```python
from build123d import *

# Parameters (mm, degrees)
F2_DEPTH    = 80
F3_DEPTH    = 5
F4_W        = 80
F4_H        = 3
F5_DEPTH    = 5
F6_T1_DEPTH = 89.0924813444
F6_T4_ANGLE = 180
F6_T6_ANGLE = 180
F7_T1_DEPTH = 89.0924813444
F7_T4_ANGLE = 180
F7_T6_ANGLE = 180


# Not quite as in the source:
# - a fillet or chamfer that OpenCascade refuses, or shapes differently, is made with other operations: its cross-section is extruded or revolved along the edge and cut away or added


with BuildPart() as f2:
    # F0 (on Top) → F2 (new body)
    with BuildSketch(Plane.XY):
        with BuildLine():
            Line((44.6416767532, 25), (-44.4508045912, 25))
            ThreePointArc((-44.4508045912, 25), (-69.4508045912, 0), (-44.4508045912, -25))
            Line((-44.4508045912, -25), (44.6416767532, -25))
            ThreePointArc((44.6416767532, -25), (69.6416767532, 0), (44.6416767532, 25))
        make_face()
        with BuildLine():
            Line((-45.3583232468, 19.9793996379), (-45.3583232468, 20.0206003621))
            Line((-45.3583232468, 20.0206003621), (44.6416767532, 20.0206003621))
            Line((44.6416767532, 20.0206003621), (44.6416767532, 20))
            ThreePointArc((44.6416767532, 20), (64.6365259994, -0.4538762181), (43.7341580975, -19.9793996379))
            Line((43.7341580975, -19.9793996379), (-43.5432859355, -19.9793996379))
            ThreePointArc((-43.5432859355, -19.9793996379), (-44.4508045912, -20), (-45.3583232468, -19.9793996379))
            ThreePointArc((-45.3583232468, -19.9793996379), (-64.4508045912, 0), (-45.3583232468, 19.9793996379))
        make_face(mode=Mode.SUBTRACT)
    extrude(amount=F2_DEPTH)

    # F1 (on Top) → F3 (join)
    with BuildSketch(Plane.XY):
        with BuildLine():
            Line((45.1049394906, 20), (-44.8950605094, 20))
            ThreePointArc((-44.8950605094, 20), (-64.8950605094, 0), (-44.8950605094, -20))
            Line((-44.8950605094, -20), (-39.8680716753, -20))
            Line((-39.8680716753, -20), (40.1319283247, -20))
            Line((40.1319283247, -20), (45.1049394906, -20))
            ThreePointArc((45.1049394906, -20), (65.1049394906, 0), (45.1049394906, 20))
        make_face()
    extrude(amount=F3_DEPTH)

    # F4 (on face) → F5 (join)
    with BuildSketch(Plane.XY.offset(5)):
        with Locations((0.1319283247, -1.5)):
            Rectangle(F4_W, F4_H)
    extrude(amount=F5_DEPTH)

    # F6: fillet of radius 5 on 1 edges, made by hand

    # F6_s2 → F6_t1 (cut)
    with BuildSketch(Plane.YZ.offset(-44.4508045912)):
        with BuildLine():
            ThreePointArc((-20, 80), (-23.5355339059, 78.5355339059), (-25, 75))
            Line((-25, 75), (-25, 80))
            Line((-25, 80), (-20, 80))
        make_face()
        with BuildLine():
            ThreePointArc((25, 75), (23.5355339059, 78.5355339059), (20, 80))
            Line((20, 80), (25, 80))
            Line((25, 80), (25, 75))
        make_face()
    extrude(amount=F6_T1_DEPTH, mode=Mode.SUBTRACT)

    # F6_s3 → F6_t4 (revolve, cut)
    with BuildSketch(Plane.YZ.offset(-44.4508045912)):
        with BuildLine():
            ThreePointArc((25, 75), (23.5355339059, 78.5355339059), (20, 80))
            Line((20, 80), (25, 80))
            Line((25, 80), (25, 75))
        make_face()
    revolve(axis=Axis((-44.4508045912, 0, 80), (0, 0, 1)), revolution_arc=F6_T4_ANGLE, mode=Mode.SUBTRACT)

    # F6_s5 → F6_t6 (revolve, cut)
    with BuildSketch(Plane.YZ.offset(44.6416767532)):
        with BuildLine():
            ThreePointArc((-25, 75), (-23.5355339059, 78.5355339059), (-20, 80))
            Line((-20, 80), (-25, 80))
            Line((-25, 80), (-25, 75))
        make_face()
    revolve(axis=Axis((44.6416767532, 0, 80), (0, 0, 1)), revolution_arc=F6_T6_ANGLE, mode=Mode.SUBTRACT)

    # F7: fillet of radius 5 on 5 edges, made by hand

    # F7_s2 → F7_t1 (cut)
    with BuildSketch(Plane.YZ.offset(-44.4508045912)):
        with BuildLine():
            ThreePointArc((-20, 0), (-23.5355339059, 1.4644660941), (-25, 5))
            Line((-25, 5), (-25, 0))
            Line((-25, 0), (-20, 0))
        make_face()
        with BuildLine():
            ThreePointArc((25, 5), (23.5355339059, 1.4644660941), (20, 0))
            Line((20, 0), (25, 0))
            Line((25, 0), (25, 5))
        make_face()
    extrude(amount=F7_T1_DEPTH, mode=Mode.SUBTRACT)

    # F7_s3 → F7_t4 (revolve, cut)
    with BuildSketch(Plane.YZ.offset(-44.4508045912)):
        with BuildLine():
            ThreePointArc((20, 0), (23.5355339059, 1.4644660941), (25, 5))
            Line((25, 5), (25, 0))
            Line((25, 0), (20, 0))
        make_face()
    revolve(axis=Axis((-44.4508045912, 0, 0), (0, 0, 1)), revolution_arc=F7_T4_ANGLE, mode=Mode.SUBTRACT)

    # F7_s5 → F7_t6 (revolve, cut)
    with BuildSketch(Plane.YZ.offset(44.6416767532)):
        with BuildLine():
            ThreePointArc((-20, 0), (-23.5355339059, 1.4644660941), (-25, 5))
            Line((-25, 5), (-25, 0))
            Line((-25, 0), (-20, 0))
        make_face()
    revolve(axis=Axis((44.6416767532, 0, 0), (0, 0, 1)), revolution_arc=F7_T6_ANGLE, mode=Mode.SUBTRACT)


solid = f2.part
```
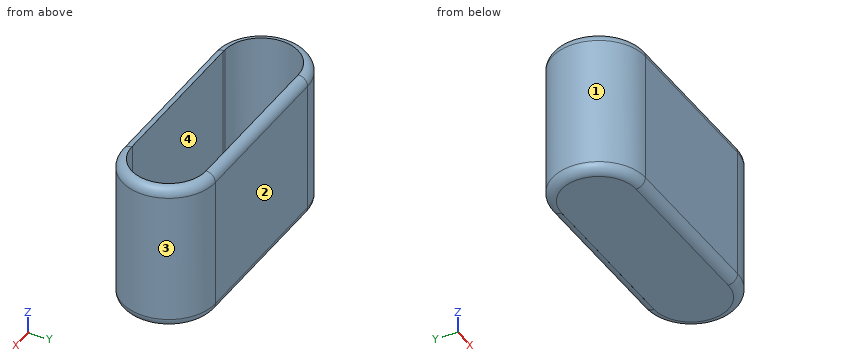
Geometry check sheet. Reference: the model listing, model coordinates, mm. Face numbers are marked on the shaded views. Coordinates: 2 decimals unless noted, no trailing zeros. Answer as a JSON object with one key per item and string values.
Q1. Scan lines: line 1 (Y direction, x = -32, z = 17.5); line 2 (Z direction, x = 12, y = -8.5); line 3 (X direction, y = -1, z = 62.5). Record each from-to range of solid material in increasing order.
Results are:
{"line 1": "y = -25 to -19.98, 20.02 to 25", "line 2": "z = 0 to 5", "line 3": "x = -69.43 to -64.43, 64.62 to 69.62"}
Q2. Depth check by flat-ended pin: pin 1 Ø5 at (y, z) = (14, 71) entering from -X; pin 2 Ø10 at (y, z) = (18, 22.5) entering from +X; pin 3 Ø2 at (y, z) = (-8.5, 44.5) entering from +X; pin 4 Ø5 at (x, z) = (46.5, 33) entering from -Y. Enter the tip coordinate at first touch or a pass-through.
Results are:
{"pin 1": "stops at x = -66.65", "pin 2": "stops at x = 66", "pin 3": "stops at x = 68.49", "pin 4": "stops at y = -25"}
Q3. Release check for a two-part mould opening along X. For the marked faces 1, 2, 3 and 4 record: released by +X, released by -X, zero draft, split by the parting line, or undercut.
Results are:
{"face 1": "released by -X", "face 2": "zero draft", "face 3": "released by +X", "face 4": "undercut"}
